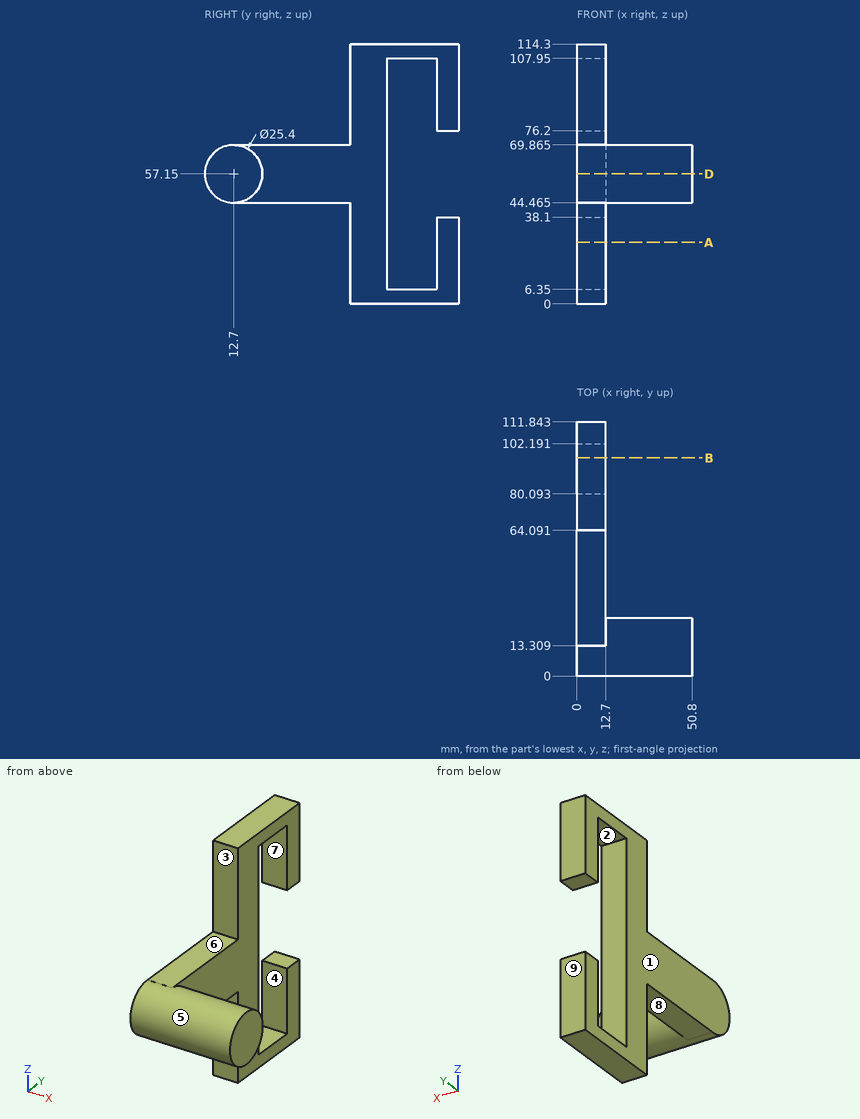
For this review, use the dimensioned drawing (mm, ordinates from the lowest corner) and the shaded views. A direction names the side the tool comes from. Give positions to 0.01 mm unless a question says otherwise; leave off trailing zeros. Loops run counter-clockwise (first coordinate to the right, second up) from the corner with the lowest first, then second, coordinate; pieces in that order, holes last. Notation, with made-up numbers: (48, 34) -> (84, 34) arc R10 ccw to (84, 48) -> close; hole circle Ø4 at (-4.5, 3.5). An arc over 180 degrees is marked (long way). One line per question, with ' | ' between items. Start each with the question number.
(1) We need section A-A (z = 27). State the section outline as (x, y) points.
(2) We need section B-B (y = 96). State the section outline as (x, z) points, and give its area (3 significant figures).
(3) For the marked faces 5, 6, 7, 8 and 9, list the 3-axis set-ups (+Z, -Z, +X, -X, +Y, -Y) from which the entire face can be reached by the end or side of a thin tool; tool diameter is ignored.
(4) We need section D-D (z = 57.15). State the section outline as (x, y) points.
(5) Insertion check: P1, Ø6.5, axis at x = 7, y = 31, coming from the -Z side (1 decimal); P2, Ø4, axis at x = 5, z = 93.5, coming from the -Y side; P3, Ø10, axis at x = 6.5, y = 40, coming from the +Z side (1 decimal). Each pin has a flat end and moves straight along its axis. Give the tip position at first contact, or say it passes through.
(6) For line 1 (Y direction, x = 2, z = 85.5); line 2 (Z direction, x = 12, y = 60) (1 decimal); line 3 (X direction, y = 68.5, z = 41.5), list the stretches that pass through material, from the lowest coordinate up.
(7) Draft analysis for pull direction Y (two halves, no side actions). For the marked faces 1, 2, 3 and 4, state which applies: +Y half, -Y half, draft (parallel to the pull), parting line (faces both ways), or undercut.
The answers:
1) outline: (0, 64.09) -> (12.7, 64.09) -> (12.7, 80.09) -> (0, 80.09) -> close; (0, 102.19) -> (12.7, 102.19) -> (12.7, 111.84) -> (0, 111.84) -> close
2) outline: (0, 0) -> (12.7, 0) -> (12.7, 6.35) -> (0, 6.35) -> close; (0, 107.95) -> (12.7, 107.95) -> (12.7, 114.3) -> (0, 114.3) -> close | area: 161 mm^2
3) face 5: +X | face 6: +Z, +X, -X, -Y | face 7: +X, -X | face 8: -Z, +X, -X, -Y | face 9: +Z, -Z, +X, -X, +Y
4) outline: (0, 0) -> (50.8, 0) -> (50.8, 25.4) -> (12.7, 25.4) -> (12.7, 80.09) -> (0, 80.09) -> close
5) P1: stops at z = 44.5 | P2: stops at y = 64.09 | P3: stops at z = 69.9
6) line 1: y = 64.09 to 80.09, 102.19 to 111.84 | line 2: z = 44.5 to 69.9 | line 3: x = 0 to 12.7
7) face 1: draft | face 2: undercut | face 3: -Y half | face 4: undercut
